Check sheet for the modelled part. Datum: model origin and axes. Units: mm. Face numbers are marked on the shaded views. A direction names the side the tool comes from. Coordinates: 2 decimals unless noted, no trailing zeros. Write each loop counter-clockwise with the first axis right and the second up, starting at its lowest first coordinate (ties: lowest second). Pieces come first, ordered by that corner, then holes. Notation, with made-up numbers: (22, 43) - (59, 43) arc R21 ccw to (59, 79) - close; hole circle Ø7 at (47, -39.75). An arc over 180 degrees is marked (long way). Answer as CSV lines item,"result". Start each with the question number.
Autodesk Inventor part; units mm, degrees
ref_plane "YZ Plane" through (0, 0, 0) normal (1, 0, 0) x (0, 1, 0)
ref_plane "XZ Plane" through (0, 0, 0) normal (0, 1, 0) x (-1, 0, 0)
ref_plane "XY Plane" through (0, 0, 0) normal (0, 0, 1) x (1, 0, 0)
sketch "Sketch1" plane through (0, 0, 0) normal (0, 0, 1) x (1, 0, 0)
  line L0 (-5.1724, -7.3755) -> (20.2276, -7.3755)
  line L1 (20.2276, -7.3755) -> (20.2276, 5.3245)
  line L2 (20.2276, 5.3245) -> (-5.1724, 5.3245)
  line L3 (-5.1724, 5.3245) -> (-5.1724, -7.3755)
  circle A0 centre (1.1776, -2.613) radius 3.175
  circle A1 centre (13.8776, -2.613) radius 3.175
  point P0 (0, 0)
  dimension "d0" = 25.4
  dimension "d1" = 12.7
  dimension "d2" = 6.35
  dimension "d3" = 6.35
  dimension "d5" = 6.35
  dimension "d6" = 6.35
  dimension "d13" = 4.7625
  dimension "d14" = 4.7625
extrude "Extrusion1" add sketch "Sketch1" along normal blind 3.175
sketch "Sketch2" plane through (0, 0, 3.175) normal (0, 0, 1) x (1, 0, 0)
  line L0 (20.2276, 5.3245) -> (20.2276, -7.3755)
  line L1 (-5.1724, 5.3245) -> (20.2276, 5.3245)
  line L2 (-5.1724, 5.3245) -> (20.2276, 5.3245)
  line L3 (20.2276, 5.3245) -> (20.2276, 2.1495)
  line L4 (20.2276, 2.1495) -> (-5.1724, 2.1495)
  line L5 (-5.1724, 2.1495) -> (-5.1724, 5.3245)
  point P0 (0, 0)
  dimension "d10" = 3.175
extrude "Extrusion2" add sketch "Sketch2" along normal blind 22.225
sketch "Sketch3" plane through (-5.1724, 2.1495, 3.175) normal (0, -1, 0) x (1, 0, 0)
  circle A0 centre (12.7, 11.1125) radius 1.5875
  point P0 (5.1724, -3.175)
  dimension "d15" = 3.175
extrude "Extrusion3" cut sketch "Sketch3" against normal blind 22.225
fillet "Fillet1" radius 3.175 4 edges at (20.2276, 3.737, 25.4) (-5.1724, 3.737, 25.4) (20.2276, -7.3755, 1.5875) (-5.1724, -7.3755, 1.5875)
equation "\"d3\" = d2"
equation "\"d14\" = d13"
properties part number "Shooter Curve Support"
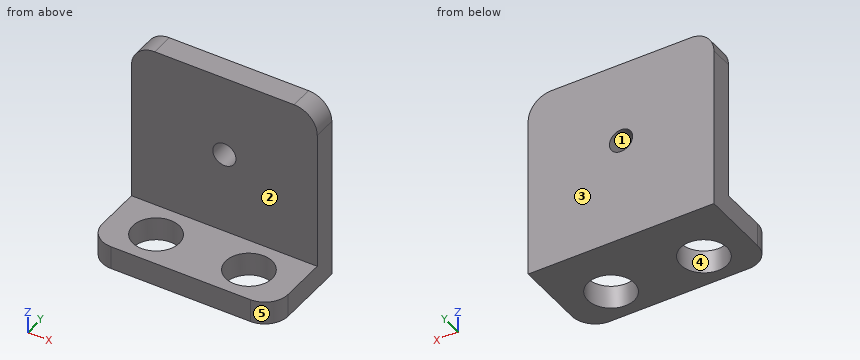
(1) Material ranges on probe 1 along Z at (x, y) = (9.5, -2.75) (3 decimals); probe 2 along Y at (x, z) = (13, 6.75); probe 3 along Y at (x, z) = (0.5, 2.5), recorded low to high. Write a range as from..to.
(2) Tool access check on the marked faces 1 and 2. Record the directions out of +Z, -Z, +X, -X, +Y, -Y that give a thin tool (end or side, any length) a straight path to the whole face; none if there is none.
(3) Cross-section at B-B on x = 12. Record the boundary of the cut face in (y, z) (1 decimal), plus the area to 3 significant figures.
(4) Release check for a two-part mould opening along X. For the marked faces 3, 4 and 5 record: pulls with the +X half, pulls with the -X half, needs draft (parallel to the pull), parting line crosses it, or undercut.
(5) Cross-section at C-C on y = -1.5. Record the boundary of the cut face in (x, z) (3 decimals).
(6) Cross-section at A-A on z = 13.5. Record the boundary of the cut face in (x, y), plus the area to 3 significant figures.
(7) Go/stop test with flat-tipped pins: P1, Ø4, axis at x = 16, z = 18, coming from the -Y side; P2, Ø6, axis at x = 16.5, y = -2, coming from the +Z side (3 decimals). Record where each tip stops, or that it passes through.
Checked values:
1,probe 1,"0..3.175"
1,probe 2,"2.15..5.32"
1,probe 3,"-7.38..-5.71, 0.49..5.32"
2,face 1,"+Y, -Y"
2,face 2,"+Z, +X, -X, -Y"
3,outline,"(-7.4, 0) - (-5.2, 0) - (-5.2, 3.2) - (-7.4, 3.2) - close; (-0.1, 0) - (5.3, 0) - (5.3, 25.4) - (2.1, 25.4) - (2.1, 3.2) - (-0.1, 3.2) - close"
3,area,"94.6 mm^2"
4,face 3,"needs draft"
4,face 4,"undercut"
4,face 5,"pulls with the +X half"
5,outline,"(-5.172, 0) - (-1.796, 0) - (-1.796, 3.175) - (-5.172, 3.175) - close; (4.151, 0) - (10.904, 0) - (10.904, 3.175) - (4.151, 3.175) - close; (16.851, 0) - (20.228, 0) - (20.228, 3.175) - (16.851, 3.175) - close"
6,outline,"(-5.17, 2.15) - (6.15, 2.15) - (6.15, 5.32) - (-5.17, 5.32) - close; (8.91, 2.15) - (20.23, 2.15) - (20.23, 5.32) - (8.91, 5.32) - close"
6,area,"71.9 mm^2"
7,P1,"y = 2.15"
7,P2,"z = 3.175"
